from build123d import *

# Parameters (mm, degrees)
SKETCH1_R           = 7
BOSS_EXTRUDE1_DEPTH = 44
SKETCH70_W          = 24
SKETCH70_H          = 39.803664443
SKETCH71_W          = 34
SKETCH71_H          = 19
CUT_EXTRUDE1_DEPTH  = 43
SKETCH73_R          = 5.5
CUT_EXTRUDE3_DEPTH  = 99.478424033
SKETCH75_W          = 19
SKETCH75_H          = 19
CUT_EXTRUDE4_DEPTH  = 105.177732746


with BuildPart() as part:
    # Sketch1 → Boss-Extrude1 (new body)
    with BuildSketch(Plane.XY):
        with BuildLine():
            Line((0, 0), (-7, 7))
            Line((-7, 7), (-7, 25))
            Line((-7, 25), (0, 32))
            Line((0, 32), (6.423127039, 32))
            Line((6.423127039, 32), (29.319429923, 27.962764043))
            ThreePointArc((29.319429923, 27.962764043), (41.564716358, 29.911963462), (50, 39))
            Line((50, 39), (74, 39))
            Line((74, 39), (79, 34))
            Line((79, 34), (79, 15))
            Line((79, 15), (50, -19))
            Line((50, -19), (44.788067397, -19))
            ThreePointArc((44.788067397, -19), (40.27095427, -12.128573817), (37.89327269, -4.256633834))
            ThreePointArc((37.89327269, -4.256633834), (36.210984968, -1.21075002), (32.948840798, 0))
            Line((32.948840798, 0), (0, 0))
        make_face()
        with Locations((7, 14)):
            Circle(SKETCH1_R, mode=Mode.SUBTRACT)
    extrude(amount=BOSS_EXTRUDE1_DEPTH)

    # Sketch70 → Cut-Revolve3 (revolve, cut)
    with BuildSketch(Plane(origin=(79, 0, 0), x_dir=(0, 0, -1), z_dir=(1, 0, 0))):
        with Locations((-24, 19.098167778)):
            Rectangle(SKETCH70_W, SKETCH70_H)
    revolve(axis=Axis((79, 39, 36), (0, 0, -1)), mode=Mode.SUBTRACT)

    # Sketch71 → Cut-Extrude1 (cut)
    with BuildSketch(Plane(origin=(0, 39, 0), x_dir=(1, 0, 0), z_dir=(0, 1, 0))):
        with Locations((10, -34.5)):
            Rectangle(SKETCH71_W, SKETCH71_H)
    extrude(amount=-CUT_EXTRUDE1_DEPTH, mode=Mode.SUBTRACT)

    # Sketch73 → Cut-Extrude3 (cut, through all)
    with BuildSketch(Plane.XY):
        with Locations(Location((65, 25, 0), (0, 0, 180))):
            Circle(SKETCH73_R)
    extrude(amount=CUT_EXTRUDE3_DEPTH, mode=Mode.SUBTRACT)

    # Sketch75 → Cut-Extrude4 (cut, through all)
    with BuildSketch(Plane(origin=(79, 0, 0), x_dir=(0, 0, -1), z_dir=(1, 0, 0))):
        with Locations((-34.5, -9.5)):
            Rectangle(SKETCH75_W, SKETCH75_H)
    extrude(amount=-CUT_EXTRUDE4_DEPTH, mode=Mode.SUBTRACT)


solid = part.part
Verification items for the finished model (mm, model axes). A direction names the side the tool comes from. Give positions to 0.01 mm unless a question says otherwise; leave off trailing zeros. Write each loop counter-clockwise with the first axis right and the second up, starting at its lowest first coordinate (ties: lowest second). Pieces come first, ordered by that corner, then holes.
(1) Gauge pin test, flat ends, axial feed: pin 1 (22.5 mm diameter, centred on x = 7, y = 14, fed in from +Z); pin 2 (1.9 mm diameter, centred on x = 3, z = 13.5, fed in from +Y); pin 3 (2 mm diameter, centred on y = -12.5, z = 14.5, fed in from -X). Record the tip position at first contact, or that the pin passes through.
(2) Cross-section at C-C (x = 65). Enter the section's corners in (y, z).
(3) Mould release check, pull along Z, two halves, no side actions. Record for faces 1 (the face through (59, 20, 36)), 2 (the face through (53, 20, 44)), 3 (the face through (79, 25, 6)): +Z half, -Z half, draft (parallel to the pull), parting line (faces both ways), or undercut.
(4) Material ranges on line 1 (Z direction, x = 69.5, y = 5); line 2 (Y direction, x = 65, z = 41); line 3 (X direction, y = 25, z = 7.5), recorded low to high.
(5) Access from +Z, -Z, +X, -X, +Y, -Y to the whole of each face (thin tool, end or side, straight path). Record for faces 4 (the face through (50.234, 11.489, 23.832)), 5 (the face through (27, 14, 35)), 6 (the face through (-3, 3, 12)).
(6) Cross-section at A-A (z = 22). Enter the section's corners in (x, y).
(7) Cross-section at B-B (y = 22). Enter the section's corners in (x, z), plus the area to 3 significant figures.
(8) Cross-section at D-D (z = 3). Enter the section's corners in (x, y).
Worked out:
1. pin 1: stops at z = 25
1. pin 2: stops at y = 32
1. pin 3: stops at x = 39.99
2. outline: (-1.41, 0) - (19.5, 0) - (19.5, 12) - (1.74, 12) - (1.74, 36) - (19.5, 36) - (19.5, 44) - (0, 44) - (0, 25) - (-1.41, 25) - close; (30.5, 0) - (39, 0) - (39, 12) - (30.5, 12) - close; (30.5, 36) - (39, 36) - (39, 44) - (30.5, 44) - close
3. face 1: undercut
3. face 2: +Z half
3. face 3: draft
4. line 1: z = 0 to 12, 36 to 44
4. line 2: y = 0 to 19.5, 30.5 to 39
4. line 3: x = -7 to 59.5, 70.5 to 79
5. face 4: +X, +Y
5. face 5: +Z, -X, +Y, -Y
5. face 6: +Z, -Z, -X, -Y
6. outline: (-7, 7) - (0, 0) - (32.95, 0) arc R5 cw to (37.89, -4.26) arc R28.63 ccw to (44.79, -19) - (50, -19) - (67.08, 1.02) arc R39.8 cw to (40.39, 29.33) arc R19 cw to (29.32, 27.96) - (6.42, 32) - (0, 32) - (-7, 25) - close; hole circle Ø14 at (7, 14)
7. outline: (-7, 0) - (60.39, 0) - (60.39, 12) - (43.01, 12) - (43.01, 36) - (60.39, 36) - (60.39, 44) - (27, 44) - (27, 25) - (-7, 25) - close; (69.61, 0) - (79, 0) - (79, 12) - (69.61, 12) - close; (69.61, 36) - (79, 36) - (79, 44) - (69.61, 44) - close
7. area: 2,090 mm2
8. outline: (-7, 7) - (0, 0) - (32.95, 0) arc R5 cw to (37.89, -4.26) arc R28.63 ccw to (44.79, -19) - (50, -19) - (79, 15) - (79, 34) - (74, 39) - (50, 39) arc R19 cw to (29.32, 27.96) - (6.42, 32) - (0, 32) - (-7, 25) - close; hole circle Ø14 at (7, 14); hole circle Ø11 at (65, 25)
